Can you work these out from the model? Positions are in its coordinate system, mm. A direction names the side the tool comes from. Round coordinates to 2 decimals unless told otherwise and drop trailing zeros. Write each loop counter-clockwise with the first axis right and the second up, starting at its lowest first coordinate (ties: lowest second). Pieces come first, ordered by that corner, then holes. Notation, with made-up numbers: (84.5, 6.5) - (98.5, 6.5) arc R8 cw to (98.5, 14.5) - close; hole circle Ø8 at (-7, 55.5). An arc over 180 degrees is marked (long way). One line per item, written item: value. Start each with the question number.
(1) I want a section at A-A on x = -85. List the corners of the cut face in (y, z) for me.
(2) On a 3-axis mill with a long thin cutter (end or side, diameter ignored), from which of +Z, -Z, +X, -X, +Y, -Y can I reach the whole of each face in a straight line? I mean faces 4 (the face through (-120, 5, -25)), 5 (the face through (-2.465, 5.121, -32.253)). Say none if no direction works.
(3) If I drill on L1, parallel to X at y = 5.25, z = -20; L2, parallel to Y at x = -3.7, z = -35; L3, parallel to Z at x = -105, y = 5.25, over which ranges is the centre line in solid material (lowest first)? Write a range as from..to.
(4) I want a section at B-B on z = -25. List the corners of the cut face in (x, y) for me.
(5) Thinking about a two-plate mould opening in X: for faces 1 (the face through (-2.465, 3.327, -12.818)), 2 (the face through (-107.747, 5.07, -20.121)), 3 (the face through (0, 5, -25)), which applies, +X half, -X half, draft (parallel to the pull), parting line (faces both ways), or undercut?
(6) I want a section at D-D on z = -20. List the corners of the cut face in (x, y) for me, plus the area to 3 significant figures.
(7) I'm going to push flat-ended pins straight in: pin 1 Ø4.5 at (x, z) = (-85, -20) entering from -Y; pin 2 Ø1.6 at (y, z) = (5, -35.5) entering from +X. Where does each tip first touch, or does it pass through?
(8) I want a section at C-C on y = 5. List the corners of the cut face in (x, z) for me, plus the area to 3 significant figures.
Autodesk Inventor part; units mm, degrees
ref_plane "YZ Plane" through (0, 0, 0) normal (1, 0, 0) x (0, 1, 0)
ref_plane "XZ Plane" through (0, 0, 0) normal (0, 1, 0) x (-1, 0, 0)
ref_plane "XY Plane" through (0, 0, 0) normal (0, 0, 1) x (1, 0, 0)
sketch "Sketch1" plane through (0, 0, 0) normal (0, 1, 0) x (-1, 0, 0)
  line L0 (0, 0) -> (120, 0)
  line L1 (120, 0) -> (120, -50)
  line L2 (120, -50) -> (0, -50)
  line L3 (0, -50) -> (0, 0)
  circle A0 centre (30, -25) radius 14
  dimension "d0" = 120
  dimension "d1" = 50
  dimension "d4" = 28
  dimension "d5" = 30
extrude "Extrusion2" add sketch "Sketch1" along normal blind 10
sketch "Sketch2" plane through (0, 10, 0) normal (0, 1, 0) x (1, 0, 0)
  circle A0 centre (-105, 20) radius 2.75
  line L0 (-120, 50) -> (-120, 0)
  line L1 (0, 50) -> (-120, 50)
  circle A1 centre (-85, 20) radius 2.75
  line L2 (-120, 0) -> (0, 0)
  dimension "d8" = 5.5
  dimension "d9" = 50
  dimension "d11" = 15
  dimension "d14" = 20
  dimension "d21" = 20
extrude "Extrusion3" cut sketch "Sketch2" against normal blind 10
sketch "Sketch3" plane through (0, 0, 0) normal (1, 0, 0) x (0, 0, -1)
  circle A0 centre (15, 5) radius 2.75
  line L0 (0, 10) -> (50, 10)
  line L1 (0, 0) -> (0, 10)
  circle A1 centre (35, 5) radius 2.75
  dimension "d22" = 5.5
  dimension "d23" = 10
  dimension "d24" = 50
  dimension "d25" = 5
  dimension "d28" = 20
  dimension "d33" = 15
extrude "Extrusion4" cut sketch "Sketch3" against normal blind 5
equation "\"d25\" = 0.5 * d23"
equation "\"d33\" = -0.5 * d28 + 0.5 * d24"
properties part number "DriverElevatorConnection" material "Steel, Carbon"
Established:
1. outline: (0, -50) - (10, -50) - (10, -22.75) - (0, -22.75) - close; (0, -17.25) - (10, -17.25) - (10, 0) - (0, 0) - close
2. face 4: +Z, -Z, -X, +Y, -Y
2. face 5: +X
3. L1: -120..-107.75, -102.25..-87.75, -82.25..-43.08, -16.92..0
3. L2: 0..2.25, 7.75..10
3. L3: -50..-22.75, -17.25..0
4. outline: (-120, 0) - (-44, 0) - (-44, 10) - (-120, 10) - close; (-16, 0) - (0, 0) - (0, 10) - (-16, 10) - close
5. face 1: draft
5. face 2: undercut
5. face 3: +X half
6. outline: (-120, 0) - (-107.75, 0) - (-107.75, 10) - (-120, 10) - close; (-102.25, 0) - (-87.75, 0) - (-87.75, 10) - (-102.25, 10) - close; (-82.25, 0) - (-43.08, 0) - (-43.08, 10) - (-82.25, 10) - close; (-16.92, 0) - (0, 0) - (0, 10) - (-16.92, 10) - close
6. area: 828 mm2
7. pin 1: through
7. pin 2: x = -5
8. outline: (-120, -50) - (0, -50) - (0, -37.75) - (-5, -37.75) - (-5, -32.25) - (0, -32.25) - (0, -17.75) - (-5, -17.75) - (-5, -12.25) - (0, -12.25) - (0, 0) - (-120, 0) - close; hole circle Ø5.5 at (-105, -20); hole circle Ø5.5 at (-85, -20); hole circle Ø28 at (-30, -25)
8. area: 5,280 mm2
